Work out the finished part from the listing and answer in its coordinate system (mm). Face numbers are marked on the shaded views. A direction names the side the tool comes from. Round coordinates to 2 decimals unless told otherwise and drop trailing zeros. Write each loop counter-clockwise with the first axis right and the second up, starting at its lowest first coordinate (ties: lowest second). Pieces come first, ordered by that corner, then holes.
1. Find section A-A (y = 31). Write down the section's boundary in (x, z), and give its area (3 significant figures).
2. Determine the mould class of the marked faces 1, 2, 3 and 4 for opening direction Z: pulls with the +Z half, pulls with the -Z half, needs draft (parallel to the pull), parting line crosses it, or undercut.
3. A tool of negligible diameter and unlimited length cuts with its end or side. For the marked faces 5, 6, 7 and 8, from which of +Z, -Z, +X, -X, +Y, -Y can it reach the whole face along a straight path? Write none if from no direction.
4. Find section B-B (z = -33). Write down the section's boundary in (x, y), and give its area (3 significant figures).
5. Find section D-D (y = 5.5). Write down the section's boundary in (x, z), and give its area (3 significant figures).
6. Straight lines are drawn through the part: probe 1 along Z at (x, y) = (55, 4); probe 2 along X at (y, z) = (32.5, -23); probe 3 along Z at (x, y) = (60.5, 20.5). For each, find the intervals that lie inside material, in ascending order.
7. Find section C-C (x = 55). Write down the section's boundary in (y, z), and give its area (3 significant figures).
8. Flat-ended cylindrical pins translate along their axes: pin 1 Ø11 at (x, z) = (47, -37) entering from +Y; pin 2 Ø10 at (x, y) = (51, 16) entering from +Z; pin 3 Ø10 at (y, z) = (19.5, -7) entering from +X; pin 4 Ø8 at (x, z) = (55, -15) entering from -Y. Find the tip coordinate at first contact, or state that the pin passes through.
```python
from build123d import *

# Parameters (mm, degrees)
BOSS_EXTRUDE1_DEPTH            = 40
SKETCH2_W                      = 40
SKETCH2_H                      = 30
BOSS_EXTRUDE2_DEPTH            = 20
BOSS_EXTRUDE3_DEPTH            = 30
CUT_EXTRUDE1_DEPTH             = 30
SKETCH5_W                      = 70
SKETCH5_H                      = 40
BOSS_EXTRUDE4_DEPTH            = 10
SKETCH6_W                      = 20
SKETCH6_H                      = 20
CUT_EXTRUDE2_DEPTH             = 41
F_10_0_10_DIAMETER_HOLE1_D     = 10
F_10_0_10_DIAMETER_HOLE1_DEPTH = 40
FILLET1_R                      = 20


with BuildPart() as part:
    # Sketch1 → Boss-Extrude1 (new body)
    with BuildSketch(Plane(origin=(0, 0, 0), x_dir=(0, -1, 0), z_dir=(-1, 0, 0))):
        Polygon((-10, -6), (-40, -20), (-10, -20), align=None)
    extrude(amount=-BOSS_EXTRUDE1_DEPTH)

    # Sketch2 → Boss-Extrude2 (add)
    with BuildSketch(Plane(origin=(0, 0, -20), x_dir=(-1, 0, 0), z_dir=(0, 0, -1))):
        with Locations((-20, 25)):
            Rectangle(SKETCH2_W, SKETCH2_H)
    extrude(amount=BOSS_EXTRUDE2_DEPTH)

    # Sketch3 → Boss-Extrude3 (add)
    with BuildSketch(Plane(origin=(40, 0, 0), x_dir=(0, 0, -1), z_dir=(1, 0, 0))):
        Polygon((40, 10), (0, 10), (20, 40), (40, 40), align=None)
    extrude(amount=BOSS_EXTRUDE3_DEPTH)

    # Sketch4 → Cut-Extrude1 (cut)
    with BuildSketch(Plane(origin=(70, 0, 0), x_dir=(0, 0, -1), z_dir=(1, 0, 0))):
        Polygon((20, 40), (0, 10), (30, 10), (30, 30), (40, 30), (40, 40), align=None)
    extrude(amount=-CUT_EXTRUDE1_DEPTH, mode=Mode.SUBTRACT)

    # Sketch5 → Boss-Extrude4 (add)
    with BuildSketch(Plane.XZ.offset(-10)):
        with Locations((35, -20)):
            Rectangle(SKETCH5_W, SKETCH5_H)
    extrude(amount=BOSS_EXTRUDE4_DEPTH)

    # Sketch6 → Cut-Extrude2 (cut, through all)
    with BuildSketch(Plane(origin=(0, 0, -40), x_dir=(-1, 0, 0), z_dir=(0, 0, -1))):
        with Locations((-20, 30)):
            Rectangle(SKETCH6_W, SKETCH6_H)
    extrude(amount=-CUT_EXTRUDE2_DEPTH, mode=Mode.SUBTRACT)

    # Ø10.0 (10) Diameter Hole1
    with Locations(Plane(origin=(0, 0, 0), x_dir=(-1, 0, 0), z_dir=(0, -1, 0))):
        with Locations((-55, 15)):
            Hole(F_10_0_10_DIAMETER_HOLE1_D / 2, depth=F_10_0_10_DIAMETER_HOLE1_DEPTH)

    # Fillet1
    fillet1_edges = [part.edges().sort_by_distance(p)[0] for p in [
        (70, 30, -35),
    ]]
    fillet(fillet1_edges, radius=FILLET1_R)


solid = part.part
```
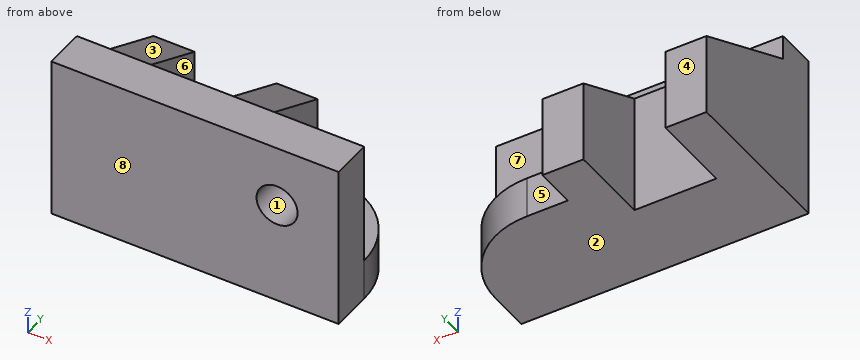
Worked answers:
1. outline: (0, -40) - (10, -40) - (10, -15.8) - (0, -15.8) - close; (30, -40) - (40, -40) - (40, -15.8) - (30, -15.8) - close
1. area: 484 mm2
2. face 1: undercut
2. face 2: pulls with the -Z half
2. face 3: pulls with the +Z half
2. face 4: needs draft
3. face 5: +Z, -Z, +X, +Y
3. face 6: +Z, -Z, +Y
3. face 7: +Z, +X, +Y
3. face 8: +Z, -Z, +X, -X, -Y
4. outline: (0, 0) - (70, 0) - (70, 10) arc R20 ccw to (50, 30) - (40, 30) - (40, 40) - (30, 40) - (30, 20) - (10, 20) - (10, 40) - (0, 40) - close
4. area: 2,010 mm2
5. outline: (0, -40) - (70, -40) - (70, 0) - (0, 0) - close; hole circle Ø10 at (55, -15)
5. area: 2,720 mm2
6. probe 1: z = -40 to -20, -10 to 0
6. probe 2: x = 0 to 10, 30 to 40
6. probe 3: z = -40 to -30
7. outline: (0, -40) - (29.36, -40) - (29.36, -30) - (10, -30) - (10, -20) - (0, -20) - close; (0, -10) - (10, -10) - (10, 0) - (0, 0) - close
7. area: 494 mm2
8. pin 1: stops at y = 30
8. pin 2: stops at z = -30
8. pin 3: stops at x = 40
8. pin 4: passes through
